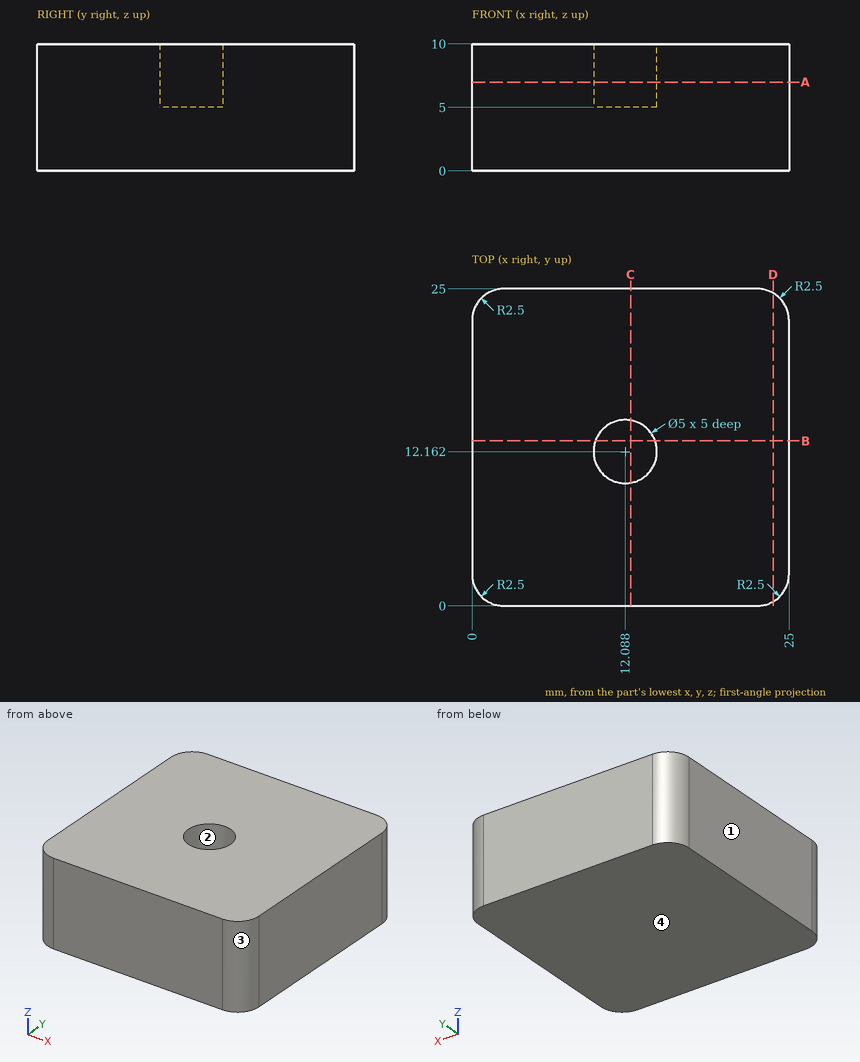
Can you work these out from the drawing? Everything is in mm from the part's minimum corner. Coordinates: 2 decimals unless noted, no trailing zeros. Write each loop counter-clockwise with the first axis right and the second up, starting at its lowest first coordinate (ties: lowest second). Pieces come first, ordered by that corner, then holes. Notation, with made-up numbers: (3.5, -35) -> (32.5, -35) arc R31 cw to (32.5, -4) -> close; hole circle Ø7 at (-13.75, -19.5). An arc over 180 degrees is marked (long way). Write each question's results on one line, items separated by ' | '. Start each with the question number.
Q1. I'm going to push a flat-ended pin straight in: pin 1 (3 mm diameter, centred on x = 12.09, y = 12.16, fed in from +Z). Where does the tip first touch, or does it pass through?
Q2. Imagine slicing it at B-B (y = 13). Write out the boundary of the cut face in (x, z).
Q3. We'd pull the mould along X, two halves only. Please class the marked faces 1, 2, 3 and 4: +X half, -X half, draft (parallel to the pull), parting line (faces both ways), or undercut.
Q4. Imagine slicing it at A-A (z = 7). Write out the boundary of the cut face in (x, y).
Q5. Imagine slicing it at C-C (x = 12.5). Write out the boundary of the cut face in (y, z) (1 decimal).
Q6. If I drill on probe 1 along Y at (x, z) = (12, 6.5); probe 2 along X at (y, z) = (13, 6.5); probe 3 along X at (y, z) = (24, 7), over which ranges is the centre line in solid material (lowest first)?
Q7. Imagine slicing it at D-D (x = 23.75). Write out the boundary of the cut face in (y, z) (1 decimal).
Taken from the geometry:
1) pin 1: stops at z = 5
2) outline: (0, 0) -> (25, 0) -> (25, 10) -> (14.44, 10) -> (14.44, 5) -> (9.73, 5) -> (9.73, 10) -> (0, 10) -> close
3) face 1: -X half | face 2: undercut | face 3: +X half | face 4: draft
4) outline: (0, 2.5) arc R2.5 ccw to (2.5, 0) -> (22.5, 0) arc R2.5 ccw to (25, 2.5) -> (25, 22.5) arc R2.5 ccw to (22.5, 25) -> (2.5, 25) arc R2.5 ccw to (0, 22.5) -> close; hole circle Ø5 at (12.09, 12.16)
5) outline: (0, 0) -> (25, 0) -> (25, 10) -> (14.6, 10) -> (14.6, 5) -> (9.7, 5) -> (9.7, 10) -> (0, 10) -> close
6) probe 1: y = 0 to 9.66, 14.66 to 25 | probe 2: x = 0 to 9.73, 14.44 to 25 | probe 3: x = 0.5 to 24.5
7) outline: (0.3, 0) -> (24.7, 0) -> (24.7, 10) -> (0.3, 10) -> close
